Autodesk Inventor part; units mm, degrees
ref_plane "Work Plane1" through (0, 18, 0) normal (0, 1, 0) x (-1, 0, 0)
ref_plane "YZ Plane" through (0, 0, 0) normal (1, 0, 0) x (0, 1, 0)
ref_plane "XY Plane" through (0, 0, 0) normal (0, 0, 1) x (1, 0, 0)
sketch "Sketch1" plane through (0, 0, 0) normal (0, 1, 0) x (-1, 0, 0)
  line L0 (0, 0) -> (80, 0) construction
  line L1 (80, 0) -> (80, 15) construction
  line L2 (80, 15) -> (0, 15) construction
  line L3 (0, 15) -> (0, 0) construction
  dimension "d0" = 80
  dimension "d1" = 15
sketch "Sketch2" plane through (0, 0, 0) normal (0, 1, 0) x (-1, 0, 0)
  line L0 (80, -20) -> (69, -20)
  line L1 (69, -20) -> (69, 20)
  line L2 (69, 20) -> (80, 20)
  line L3 (80, 20) -> (80, -20)
  line L4 (55, 0) -> (44, 0)
  line L5 (44, 0) -> (44, 20)
  line L6 (44, 20) -> (55, 20)
  line L7 (55, 20) -> (55, 0)
  line L8 (71, -18) -> (78, -18)
  line L9 (78, -18) -> (78, 18)
  line L10 (78, 18) -> (71, 18)
  line L11 (71, 18) -> (71, -18)
  line L12 (53, 2) -> (46, 2)
  line L13 (46, 2) -> (46, 18)
  line L14 (46, 18) -> (53, 18)
  line L15 (53, 18) -> (53, 2)
  dimension "d2" = 11
  dimension "d3" = 40
  dimension "d6" = 11
  dimension "d10" = 2
  dimension "d11" = 2
  dimension "d110" = 20
  dimension "d111" = 14
extrude "Extrusion1" add sketch "Sketch2" along normal blind 15
sketch "Sketch3" plane through (0, 15, 0) normal (0, 1, 0) x (1, 0, 0)
  line L0 (-69, 20) -> (-80, 20)
  line L1 (-80, 20) -> (-69, 20)
  line L2 (-69, 20) -> (-69, -20)
  line L3 (-69, -20) -> (-80, -20)
  line L4 (-80, -20) -> (-80, 20)
  line L5 (-55, -20) -> (-44, -20)
  line L6 (-44, -20) -> (-55, -20)
  line L7 (-55, -20) -> (-55, 0)
  line L8 (-55, 0) -> (-44, 0)
  line L9 (-44, 0) -> (-44, -20)
  point P0 (0, 0)
  dimension "d16" = 40
extrude "Extrusion2" add sketch "Sketch3" along normal blind 3
sketch "Sketch4" plane through (-69, 0, 20) normal (1, 0, 0) x (0, 0, -1)
  circle A0 centre (7.5, 8) radius 1.5
  line L0 (2, 0) -> (38, 0)
  line L1 (0, 0) -> (0, 18) construction
  point P0 (0, 15)
  dimension "d26" = 3
  dimension "d28" = 8
  dimension "d29" = 7.5
extrude "Extrusion3" cut sketch "Sketch4" against normal blind 3
sketch "Sketch5" plane through (-55, 0, 0) normal (-1, 0, 0) x (0, 0, 1)
  circle A0 centre (12.5, 8) radius 1.5
  line L0 (20, 0) -> (20, 18)
  line L1 (2, 0) -> (18, 0)
  point P0 (0, 0)
  point P1 (20, 15)
  dimension "d33" = 3
  dimension "d34" = 7.5
  dimension "d35" = 8
extrude "Extrusion4" cut sketch "Sketch5" against normal blind 3
ref_plane "Work Plane1" through (0, 18, 0) normal (0, 1, 0) x (-1, 0, 0)
sketch "Sketch12" plane through (0, 18, 0) normal (0, 1, 0) x (-1, 0, 0)
  line L0 (80, 20) -> (50, 20)
  line L1 (50, 20) -> (50, 12)
  line L2 (50, 12) -> (80, 12)
  line L3 (80, 12) -> (80, 20)
  line L4 (55, 8) -> (55, 0)
  dimension "d59" = 30
  dimension "d60" = 8
sketch "Sketch13" plane through (0, 18, 0) normal (0, 1, 0) x (-1, 0, 0)
  line L0 (74.3573, 0) -> (62.3573, 0)
  line L1 (62.3573, 0) -> (62.3573, 15)
  line L2 (62.3573, 15) -> (74.3573, 15)
  line L3 (74.3573, 15) -> (74.3573, 0)
  line L4 (48, 12) -> (36, 12)
  line L5 (36, 12) -> (36, 21)
  line L6 (36, 21) -> (48, 21)
  line L7 (48, 21) -> (48, 12)
  line L8 (0, 0) -> (11, 0)
  line L9 (4, 0) -> (17, 0)
  line L10 (17, 0) -> (17, 17)
  line L11 (17, 17) -> (4, 17)
  line L12 (4, 17) -> (4, 0)
  dimension "d64" = 12
  dimension "d65" = 15
  dimension "d66" = 12
  dimension "d67" = 13
  dimension "d68" = 17
extrude "Extrusion9" add sketch "Sketch13" along normal blind 2
extrude "Extrusion10" add sketch "Sketch12" along normal blind 4
sketch "Sketch14" plane through (0, 20, 0) normal (0, 1, 0) x (1, 0, 0)
  line L0 (-65, -4) -> (-41.7529, -4)
  line L1 (-41.7529, -4) -> (-41.7529, -17.4715)
  line L2 (-41.7529, -17.4715) -> (-65, -17.4715)
  line L3 (-65, -17.4715) -> (-65, -4)
  point P0 (0, 0)
extrude "Extrusion11" add sketch "Sketch14" along normal blind 4
sketch "Sketch15" plane through (0, 20, 0) normal (0, 1, 0) x (1, 0, 0)
  line L0 (-69, -15) -> (-69, 0)
  line L1 (-69, -10) -> (-17, -10)
  line L2 (-17, -10) -> (-17, 10)
  line L3 (-17, 10) -> (-69, 10)
  line L4 (-69, 10) -> (-69, -10)
  point P0 (0, 0)
  point P1 (-69, -20)
  point P2 (-69, -22)
  point P3 (-69, -20)
  dimension "d76" = 52
  dimension "d77" = 20
extrude "Extrusion12" add sketch "Sketch15" along normal blind 3
sketch "Sketch16" plane through (0, 0, 0) normal (0, 1, 0) x (-1, 0, 0)
  line L0 (69, 20) -> (80, 20)
  line L1 (80, 20) -> (80, 23)
  line L2 (69, 20) -> (69, 23)
  line L3 (69, 23) -> (74.8182, 28.4908)
  line L4 (74.8182, 28.4908) -> (80, 23)
  circle A0 centre (74.5, 23) radius 1.25
  line L5 (74.5, 23) -> (80, 23) construction
  line L6 (74.5, 23) -> (69, 23) construction
  line L7 (80, 15) -> (0, 15) construction
  line L8 (44, 20) -> (44, 23)
  line L9 (49.5, 23) -> (44, 23) construction
  circle A1 centre (49.5, 23) radius 1.25
  line L10 (55, 20) -> (55, 23)
  line L11 (49.5, 23) -> (55, 23) construction
  line L12 (49.8182, 28.4908) -> (55, 23)
  line L13 (44, 23) -> (49.8182, 28.4908)
  line L14 (55, 20) -> (44, 20)
  dimension "d80" = 3
  dimension "d81" = 3
  dimension "d82" = 8
  dimension "d83" = 2.5
  dimension "d84" = 3
  dimension "d96" = 25
extrude "Extrusion14" add sketch "Sketch16" along normal blind 3
sketch "Sketch17" plane through (0, 0, 0) normal (0, 1, 0) x (-1, 0, 0)
  line L0 (44, 21.1125) -> (0, 21.1125)
  line L1 (0, 21.1125) -> (0, -22.6665)
  line L2 (0, -22.6665) -> (44, -22.6665)
  line L3 (44, -22.6665) -> (44, 21.1125)
  line L4 (44, 0) -> (44, 20)
  line L5 (55, -0.777) -> (44, -0.777)
  line L6 (44, -0.777) -> (44, -22.6665)
  line L7 (44, -22.6665) -> (55, -22.6665)
  line L8 (55, -22.6665) -> (55, -0.777)
extrude "Extrusion15" cut sketch "Sketch17" along normal through all
sketch "Sketch18" plane through (0, 0, 0) normal (0, 1, 0) x (-1, 0, 0)
  line L0 (26.5385, -0.777) -> (55, 3.223)
  line L1 (55, 3.223) -> (55, -0.777)
  line L2 (55, -0.777) -> (26.5385, -0.777)
  line L3 (55, 23) -> (55, 0)
  line L4 (55, 0) -> (44, 0)
  line L5 (69, -20) -> (69, 23)
  line L6 (44, -0.777) -> (55, -0.777)
  point P0 (0, 0)
  point P1 (57, 20)
  point P2 (69, 20)
  dimension "d103" = 8
  dimension "d104" = 4
extrude "Extrusion16" cut sketch "Sketch18" along normal through all
equation "\"d11\" = d10"
equation "\"d81\" = d80"
equation "\"d84\" = d81"
properties part number "game-over"
Can you work these out from the model? Positions are in its coordinate system, mm. A direction names the side the tool comes from. Coordinates: 2 decimals unless noted, no trailing zeros. Loops run counter-clockwise (first coordinate to the right, second up) from the corner with the lowest first, then second, coordinate; pieces in that order, holes last.
1) Thinking about a two-plate mould opening in Y: for faces 4 (the flat face through (-50, 15, 10)), 5 (the flat face through (-57, 20, 4)), 6 (the flat face through (-55, 21, -3)), 7 (the flat face through (-55, 24, 11)), which applies, pulls with the +Y half, pulls with the -Y half, needs draft (parallel to the pull), parting line crosses it, or undercut?
2) I need wall thicknesses on probe 1 along X at (y, z) = (5.5, 7); probe 2 along X at (y, z) = (8.75, 1); probe 3 along Z at (x, y) = (-73, 10). Which ranges of each line are inside material? Lowest first, please.
3) Imagine slicing it at A-A on y = 8. List the corners of the cut face in (x, z) for me.
4) Imagine slicing it at D-D on x = -52. List the corners of the cut face in (y, z) for me, plus the area to 3 significant figures.
5) For pin 1 (3 mm diameter, centred on x = -68, z = 3, fed in from +Y); pin 2 (5 mm diameter, centred on x = -54, y = 11, fed in from -Z); pin 3 (3.5 mm diameter, centred on y = 22, z = 1.5, fed in from -X), each with a flat end and sliding along its axis, tell me the tip position at first contact or that it passes through.
6) Imagine slicing it at C-C on x = -63. List the corners of the cut face in (y, z) for me.
7) Imagine slicing it at B-B on y = 11.25. List the corners of the cut face in (x, z) for me, plus the area to 3 significant figures.
8) Which directions (+Z, -Z, +X, -X, +Y, -Y) give clear straight access to the entire face, cutting with the end or side of a thin tool? Please do faces 1 (the flat face through (-62.357, 19, 6)), 2 (the flat face through (-71.87, 1.48, 25.71)), 3 (the flat face through (-63, 18, 12)).
Completed:
1. face 4: pulls with the -Y half
1. face 5: undercut
1. face 6: needs draft
1. face 7: pulls with the +Y half
2. probe 1: x = -80 to -78, -71 to -69, -55 to -53, -46 to -44
2. probe 2: x = -80 to -78, -71 to -69
2. probe 3: z = -20 to -18, 18 to 20
3. outline: (-80, -20) - (-69, -20) - (-69, 11) - (-71, 11) - (-71, -18) - (-78, -18) - (-78, 18) - (-71, 18) - (-71, 14) - (-69, 14) - (-69, 20) - (-80, 20) - close; (-55, 3.22) - (-53, 2.94) - (-53, 11) - (-55, 11) - close; (-55, 14) - (-53, 14) - (-53, 18) - (-46, 18) - (-46, 2) - (-46.3, 2) - (-44, 1.68) - (-44, 20) - (-55, 20) - close
4. outline: (0, 18) - (15, 18) - (15, 2.8) - (18, 2.8) - (18, 12) - (20, 12) - (20, 2.8) - (23, 2.8) - (23, 4) - (24, 4) - (24, 17.47) - (22, 17.47) - (22, 20) - (3, 20) - (3, 26.18) - (0, 26.18) - close
4. area: 179 mm2
5. pin 1: stops at y = 23
5. pin 2: stops at z = 2.94
5. pin 3: stops at x = -69
6. outline: (18, 0) - (20, 0) - (20, -10) - (23, -10) - (23, 4) - (24, 4) - (24, 17.47) - (22, 17.47) - (22, 20) - (18, 20) - close
7. outline: (-80, -20) - (-69, -20) - (-69, 20) - (-80, 20) - close; (-55, 3.22) - (-53, 2.94) - (-53, 18) - (-46, 18) - (-46, 2) - (-46.3, 2) - (-44, 1.68) - (-44, 20) - (-55, 20) - close; hole (-78, -18) - (-71, -18) - (-71, 18) - (-78, 18) - close
7. area: 272 mm2
8. face 1: -Z, +X, -Y
8. face 2: +Z, +Y, -Y
8. face 3: +Z, -Z, -Y
